Can you work these out from the model? Positions are in its coordinate system, mm. A direction names the side the tool comes from. Coordinates: 2 decimals unless noted, no trailing zeros. Order: outer loops, then holes, each group sorted by start corner. A loop starts at its lowest first (then second) coordinate and runs counter-clockwise, first axis right, second up.
```python
from build123d import *

# Parameters (mm, degrees)
BASE_DEPTH               = 1
SLOT_GUIDE_FILLET_1MM_R  = 1
SIDE_WALL_1_DEPTH        = 0.65
WALL_LINK_DEPTH          = 6.24
SKETCH4_W                = 2.875
SKETCH4_H                = 6.04
LOWER_FIT_DEPTH          = 1
CUT_THROUGH_REACH        = 9.184
SKETCH5_W                = 1.5
SKETCH5_H                = 1.45
SKETCH5_H_2              = 0.625
SKETCH6_W                = 0.5
SKETCH6_H                = 0.275
CUT_THROUGH_FINISH_DEPTH = 2
REAR_INSERT_DEPTH        = 0.725


with BuildPart() as part:
    # Sketch1 → Base (new body)
    with BuildSketch(Plane(origin=(0, 0, 0), x_dir=(1, 0, 0), z_dir=(0, 1, 0))):
        Polygon((3.125, 3.77), (3.125, 0.725), (0.5, 0.725), (0.5, -0.725), (3.125, -0.725), (3.125, -3.77), (-3.125, -3.77), (-3.125, 3.77), align=None)
    extrude(amount=BASE_DEPTH)

    # Slot Guide Fillet (1mm)
    slot_guide_fillet_1mm_edges = [part.edges().sort_by_distance(p)[0] for p in [
        (1.8125, 1, 0.725),
        (0.5, 1, 0),
        (1.8125, 1, -0.725),
    ]]
    fillet(slot_guide_fillet_1mm_edges, radius=SLOT_GUIDE_FILLET_1MM_R - 0.0001)  # a hair under: the kernel refuses the full size

    # Sketch2 → Side Wall 1 (add)
    with BuildSketch(Plane(origin=(0, 0, -3.77), x_dir=(-1, 0, 0), z_dir=(0, 0, -1))):
        Polygon((3.125, 1), (0.125, 1), (2.125, 3), (4.625, 3), (4.625, 2), align=None)
    side_wall_1 = extrude(amount=-SIDE_WALL_1_DEPTH)

    # Side Wall 2: Side Wall 1 across plane
    add(side_wall_1.mirror(Plane.XY))

    # Sketch3 → Wall Link (add)
    with BuildSketch(Plane.XY.offset(-3.12)):
        Polygon((-3.125, 1), (-4.625, 2), (-4.625, 3), (-4.125, 3), (-4.125, 2.267591879), (-2.223612181, 1), align=None)
    extrude(amount=WALL_LINK_DEPTH)

    # Sketch4 → Lower Fit (add)
    with BuildSketch(Plane.XZ):
        with Locations((-0.9375, 0)):
            Rectangle(SKETCH4_W, SKETCH4_H)
    extrude(amount=LOWER_FIT_DEPTH)

    # Cut Through: up to this face of the body (flat: up to its plane)
    cut_through_end = Plane(part.part.faces().sort_by_distance((-0.9375, -1, 0))[0])
    # Sketch5 → Cut Through (cut, up to the picked face)
    with BuildSketch(Plane(origin=(0, 3, 0), x_dir=(1, 0, 0), z_dir=(0, 1, 0)), mode=Mode.PRIVATE) as cut_through_sk1:
        with Locations((-3.875, 0)):
            Rectangle(SKETCH5_W, SKETCH5_H)
    cut_through_tool1 = split(extrude(cut_through_sk1.sketch, amount=-CUT_THROUGH_REACH, mode=Mode.PRIVATE), bisect_by=cut_through_end, keep=Keep.BOTH, mode=Mode.PRIVATE)
    # Sketch5 → Cut Through (cut, up to the picked face)
    with BuildSketch(Plane(origin=(0, 3, 0), x_dir=(1, 0, 0), z_dir=(0, 1, 0)), mode=Mode.PRIVATE) as cut_through_sk2:
        with Locations((-1.375, -3.0825)):
            Rectangle(SKETCH5_W, SKETCH5_H_2)
    cut_through_tool2 = split(extrude(cut_through_sk2.sketch, amount=-CUT_THROUGH_REACH, mode=Mode.PRIVATE), bisect_by=cut_through_end, keep=Keep.BOTH, mode=Mode.PRIVATE)
    # Sketch5 → Cut Through (cut, up to the picked face)
    with BuildSketch(Plane(origin=(0, 3, 0), x_dir=(1, 0, 0), z_dir=(0, 1, 0)), mode=Mode.PRIVATE) as cut_through_sk3:
        with Locations((-1.375, 3.0825)):
            Rectangle(SKETCH5_W, SKETCH5_H_2)
    cut_through_tool3 = split(extrude(cut_through_sk3.sketch, amount=-CUT_THROUGH_REACH, mode=Mode.PRIVATE), bisect_by=cut_through_end, keep=Keep.BOTH, mode=Mode.PRIVATE)
    add(cut_through_tool1.solids().sort_by(Axis((-3.875, 3, 0), (0, -1, 0)))[0], mode=Mode.SUBTRACT)
    add(cut_through_tool2.solids().sort_by(Axis((-1.375, 3, 3.0825), (0, -1, 0)))[0], mode=Mode.SUBTRACT)
    add(cut_through_tool3.solids().sort_by(Axis((-1.375, 3, -3.0825), (0, -1, 0)))[0], mode=Mode.SUBTRACT)

    # Sketch6 → Cut Through Finish (cut)
    with BuildSketch(Plane(origin=(0, 1, 0), x_dir=(1, 0, 0), z_dir=(0, 1, 0))):
        with Locations((-0.375, 3.2575)):
            Rectangle(SKETCH6_W, SKETCH6_H)
        with Locations((-0.375, -3.2575)):
            Rectangle(SKETCH6_W, SKETCH6_H)
    extrude(amount=CUT_THROUGH_FINISH_DEPTH, mode=Mode.SUBTRACT)

    # Sketch7 → Rear Insert (add, symmetric)
    with BuildSketch(Plane.XY):
        with BuildLine():
            Line((-3.125, -3), (-2.375, -3))
            Line((-2.375, -3), (-2.375, -1))
            Line((-2.375, -1), (-2.375, 0))
            Line((-2.375, 0), (-3.125, 0))
            Line((-3.125, 0), (-3.125, -0.75))
            ThreePointArc((-3.125, -0.75), (-3.198223305, -0.926776695), (-3.375, -1))
            Line((-3.375, -1), (-4.125, -1))
            Line((-4.125, -1), (-4.125, -2))
            Line((-4.125, -2), (-3.125, -3))
        make_face()
    extrude(amount=REAR_INSERT_DEPTH, both=True)


solid = part.part
```
1. On a 3-axis mill with a long thin cutter (end or side, diameter ignored), from which of +Z, -Z, +X, -X, +Y, -Y can I reach the whole of each face in a straight line? I mean faces 4 (the flat face through (-1, -1, 0)), 5 (the flat face through (-3, -1, -0.725)), 6 (the flat face through (-1.111, 1.986, -3.585)), 7 (the flat face through (-2.765, 1.361, -0.044)), 8 (the flat face through (-4.625, 2.5, 2.2)). Say none if no direction works.
Completed:
face 4: +Z, -Z, +X, -Y
face 5: -Z, -X, -Y
face 6: +Z, -Z, +X, +Y
face 7: +X, +Y
face 8: +Z, -Z, -X, +Y, -Y
2. Please list where these lines run through material, in increasing order: probe 1 along Z at (x, y) = (-2, 2.6) (3 decimals); probe 2 along Z at (x, y) = (-3.5, 2.55); probe 3 along Y at (x, z) = (-3, -3.5).
Completed:
probe 1: z = -3.77 to -3.395, 3.395 to 3.77
probe 2: z = -3.77 to -3.12, 3.12 to 3.77
probe 3: y = 0 to 3
3. Imagine slicing it at B-B on x = -1. Please give me the cut outline in (y, z) (3 decimals), then the cut area to 3 significant figures.
Completed:
outline: (-1, -2.77) - (1, -2.77) - (1, 2.77) - (-1, 2.77) - close; (0, -3.77) - (1.875, -3.77) - (1.875, -3.395) - (0, -3.395) - close; (0, 3.395) - (1.875, 3.395) - (1.875, 3.77) - (0, 3.77) - close
area: 12.5 mm2
4. Imagine slicing it at D-D on y = 1.2. Please give me the cut outline in (x, z) (3 decimals), then the cut area to 3 significant figures.
Completed:
outline: (-3.425, -3.77) - (-0.325, -3.77) - (-0.325, -3.395) - (-2.125, -3.395) - (-2.125, -3.12) - (-2.524, -3.12) - (-2.524, 3.12) - (-2.125, 3.12) - (-2.125, 3.395) - (-0.325, 3.395) - (-0.325, 3.77) - (-3.425, 3.77) - (-3.425, 0.725) - (-3.125, 0.725) - (-3.125, -0.725) - (-3.425, -0.725) - close
area: 8.23 mm2
5. Thinking about a two-plate mould opening in Z: for faces 1 (the cylindrical face through (1.74, 0.7, 1.01)), 2 (the flat face through (-3, -1, 0.725)), 3 (the flat face through (-1.111, 1.986, 3.585)), which applies, pulls with the +Z half, pulls with the -Z half, needs draft (parallel to the pull), parting line crosses it, or undercut?
Completed:
face 1: undercut
face 2: pulls with the +Z half
face 3: needs draft
6. Imagine slicing it at C-C on z = -2. Please give me the cut outline in (x, y) (3 decimals).
Completed:
outline: (-4.625, 2) - (-3.125, 1) - (-3.125, 0) - (-2.375, 0) - (-2.375, -1) - (0.5, -1) - (0.5, 0) - (3.125, 0) - (3.125, 1) - (-2.224, 1) - (-4.125, 2.268) - (-4.125, 3) - (-4.625, 3) - close
7. I'm going to push flat-ended pins straight in: pin 1 (0.9 mm diameter, centred on x = 1, z = 1.5, fed in from -Y); pin 2 (2 mm diameter, centred on x = -0.5, z = -0.5, fed in from -Y); pin 3 (2.5 mm diameter, centred on y = 0.5, z = -0.5, fed in from -X). Where does each tip first touch, or does it pass through?
Completed:
pin 1: stops at y = 0
pin 2: stops at y = -1
pin 3: stops at x = -4.22
